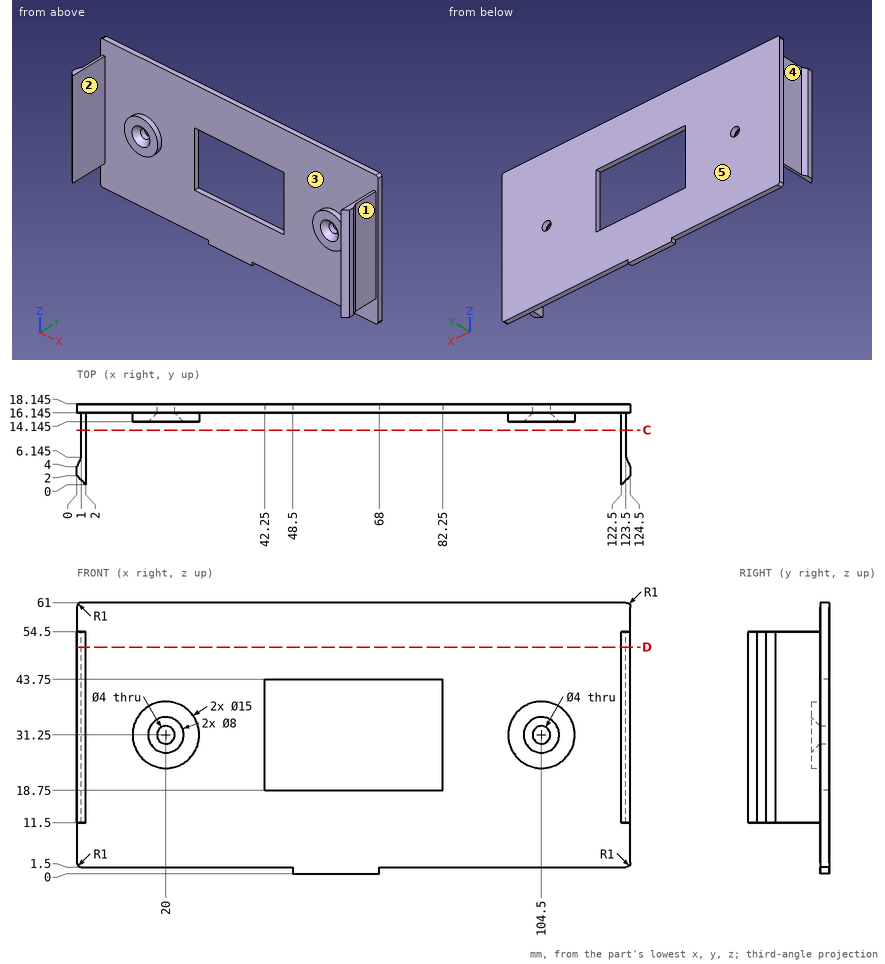
The drawing under review shows one solid part. Ordinate dimensions are in mm from its lowest x, y, z. A direction names the side the tool comes from. Give positions to 0.01 mm unless a question says otherwise; leave off trailing zeros. Loops run counter-clockwise (first coordinate to the right, second up) from the corner with the lowest first, then second, coordinate; pieces in that order, holes last. Notation, with made-up numbers: M 82.25,5 L 103.25,5 A27 ccw 103.25,38 Z; hole C 22.25,55.5 d6. An arc over 180 degrees is marked long. Return JSON: item names as keys, results as strings. Group by question number.
Item 1: Tool access review of the marked faces 1 and 2: name each direction out of +Z, -Z, +X, -X, +Y, -Y from which nothing blocks a thin tool from reaching the whole face with its end or side.
Item 2: We need section C-C (y = 12.25). Give the boundary of the cut face in (x, z).
Item 3: For probe 1 along X at (y, z) = (8.5, 16); probe 2 along X at (y, z) = (2, 47); probe 3 along Z at (x, y) = (72.5, 17.25), list the stretches that pass through material, from the lowest coordinate up.
Item 4: Insertion check: pin 1 Ø6 at (y, z) = (9, 37.5) entering from +X; pin 2 Ø5 at (y, z) = (12, 35) entering from -X; pin 3 Ø16.5 at (x, z) = (101.5, 28) entering from -Y (1 decimal). Each pin has a flat end and moves straight along its axis. Give the tip position at first contact, or say it passes through.
Item 5: Mouldability with a two-part tool opening along X and no side actions: class the marked faces 3, 4 and 5 as released by +X, released by -X, zero draft, split by the parting line, or undercut.
Item 6: We need section D-D (z = 51). Give the boundary of the cut face in (x, y) (1 decimal).
Output:
{
 "1": {"face 1": "+Z, -Z, +X", "face 2": "+Z, -Z, -Y"},
 "2": {"outline": "M 1,11.5 L 2,11.5 L 2,54.5 L 1,54.5 Z; M 122.5,11.5 L 123.5,11.5 L 123.5,54.5 L 122.5,54.5 Z"},
 "3": {"probe 1": "x = 1 to 2, 122.5 to 123.5", "probe 2": "x = 0 to 2, 122.5 to 124.5", "probe 3": "z = 1.5 to 18.75, 43.75 to 61"},
 "4": {"pin 1": "stops at x = 123.57", "pin 2": "stops at x = 1", "pin 3": "stops at y = 14.1"},
 "5": {"face 3": "undercut", "face 4": "released by -X", "face 5": "zero draft"},
 "6": {"outline": "M 0,2 L 2,0 L 2,16.1 L 122.5,16.1 L 122.5,0 L 124.5,2 L 124.5,4 L 123.5,6.1 L 123.5,16.1 L 124.5,16.1 L 124.5,18.1 L 0,18.1 L 0,16.1 L 1,16.1 L 1,6.1 L 0,4 Z"}
}
